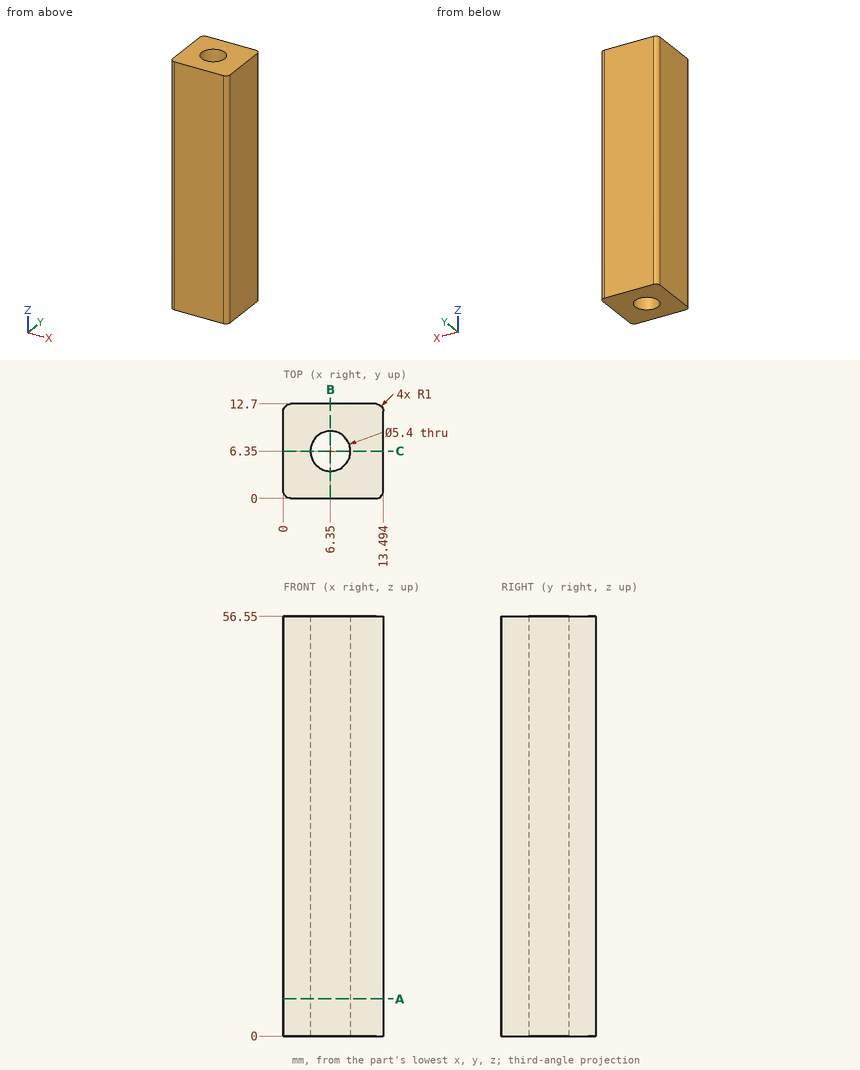
Job drawing, mm, ordinate dimensions from the low corner. One solid piece. Coordinates: 2 decimals unless noted, no trailing zeros. Order: outer loops, then holes, each group sorted by start corner. A loop starts at its lowest first (then second) coordinate and runs counter-clockwise, first axis right, second up. Notation, with made-up numbers: (20, 41) - (73, 41) arc R37 ccw to (73, 78) - close; hole circle Ø7 at (-3, 47.25). An arc over 180 degrees is marked (long way). Use CSV: the item, a comma, the result in double quotes.
Item 1: Saw through at C-C on y = 6.35. Give the cut face in (x, z), and give its area (3 significant figures).
Solved:
outline,"(0, 0) - (3.65, 0) - (3.65, 56.55) - (0, 56.55) - close; (9.05, 0) - (13.49, 0) - (13.49, 56.55) - (9.05, 56.55) - close"
area,"458 mm²"
Item 2: Saw through at B-B on x = 6.35. Give the cut face in (y, z).
Solved:
outline,"(0, 0) - (3.65, 0) - (3.65, 56.55) - (0, 56.55) - close; (9.05, 0) - (12.7, 0) - (12.7, 56.55) - (9.05, 56.55) - close"
Item 3: Probe probe 1 along Y at (x, z) = (6.35, 20.5); probe 2 along X at (y, z) = (4.25, 49) (1 decimal); probe 3 along X at (y, z) = (5.5, 42.5). List the from-to ranges inside material, lowest first.
Solved:
probe 1,"y = 0 to 3.65, 9.05 to 12.7"
probe 2,"x = 0 to 4.7, 8 to 13.5"
probe 3,"x = 0 to 3.79, 8.91 to 13.49"
Item 4: Saw through at A-A on z = 5. Give the cut face in (x, y), and give its area (3 significant figures).
Solved:
outline,"(0, 1) arc R1 ccw to (1, 0) - (12.49, 0) arc R1 ccw to (13.49, 1) - (13.49, 11.7) arc R1 ccw to (12.49, 12.7) - (1, 12.7) arc R1 ccw to (0, 11.7) - close; hole circle Ø5.4 at (6.35, 6.35)"
area,"148 mm²"
